Can you work these out from the model? Positions are in its coordinate system, mm. A direction names the side the tool comes from. Give positions to 0.01 mm unless a question says otherwise; leave off trailing zeros. Order: outer loops, then holes, each group sorted by start corner. A loop starts at its lowest first (then second) coordinate and runs counter-clockwise, first axis right, second up. Notation, with made-up numbers: (-28.5, 30.5) - (-21.5, 30.5) arc R7 cw to (-21.5, 37.5) - close; hole circle Ø8 at (17.5, -37.75). An arc over 180 degrees is marked (long way). Use one line per item in the form item = value. Start each with the question number.
1) We'd pull the mould along Y, two halves only. Please class faces 4 (the flat face through (-31.3, -1.7, 3)), 5 (the flat face through (-140.5, 83, 3)), 6 (the flat face through (-150, 86, 2)): released by +Y, released by -Y, zero draft, split by the parting line, or undercut.
2) Suppose I cut it at A-A, the plane z = 4.65. State how many separate pieces and enclosed holes the cut face has, and give its area (3 significant figures).
3) For pin 1 (3.5 mm diameter, centred on x = -30, y = -3, fed in from +Z); pin 2 (1 mm diameter, centred on x = -135, z = 1.5, fed in from -Y); pin 3 (3 mm diameter, centred on y = -4, z = 3, fed in from -X), each with a flat end and sliding along its axis, tell me the tip position at first contact or that it passes through.
4) Which directions (+Z, -Z, +X, -X, +Y, -Y) give clear straight access to the entire face, cutting with the end or side of a thin tool? Please do faces 1 (the flat face through (-20, -3, 3)), 2 (the flat face through (-40, -3, 3)), 3 (the flat face through (-269.7, 81.7, 3)).
5) Please list where these lines run through material, in increasing order: probe 1 along X at (y, z) = (83, 2.25); probe 2 along Y at (x, z) = (-150.5, 2); probe 3 along X at (y, z) = (82, 3.55).
6) Suppose I cut it at B-B, the plane x = -78.5. Write out the boundary of the cut face in (y, z), and give its area (3 significant figures).
```python
from build123d import *

# Parameters (mm, degrees)
BOSS_EXTRU_1_DEPTH      = 6
ESQUISSE2_R             = 1.5
ENL_V_MAT_EXTRU_1_DEPTH = 314.10221973
ESQUISSE3_R             = 2.995
ENL_V_MAT_EXTRU_2_DEPTH = 3


with BuildPart() as part:
    # Esquisse1 → Boss.-Extru.1 (new body)
    with BuildSketch(Plane.XY):
        Polygon((-40, 80), (-140.5, 80), (-140.5, 86), (-160.5, 86), (-160.5, 80), (-261, 80), (-261, 86), (-281, 86), (-281, 80), (-301, 80), (-301, 0), (-281, 0), (-281, -6), (-261, -6), (-261, 0), (-160.5, 0), (-160.5, -6), (-140.5, -6), (-140.5, 0), (-40, 0), (-40, -6), (-20, -6), (-20, 0), (0, 0), (0, 80), (-20, 80), (-20, 86), (-40, 86), align=None)
    extrude(amount=BOSS_EXTRU_1_DEPTH)

    # Esquisse2 → Enlèv. mat.-Extru.1 (cut, through all)
    with BuildSketch(Plane.XY.offset(6)):
        with Locations((-271, 83)):
            Circle(ESQUISSE2_R)
        with Locations((-150.5, 83)):
            Circle(ESQUISSE2_R)
        with Locations((-30, 83)):
            Circle(ESQUISSE2_R)
        with Locations(Location((-271, -3, 0), (0, 0, 180))):
            Circle(ESQUISSE2_R)
        with Locations(Location((-150.5, -3, 0), (0, 0, 180))):
            Circle(ESQUISSE2_R)
        with Locations(Location((-30, -3, 0), (0, 0, 180))):
            Circle(ESQUISSE2_R)
    extrude(amount=-ENL_V_MAT_EXTRU_1_DEPTH, mode=Mode.SUBTRACT)

    # Esquisse3 → Enlèv. mat.-Extru.2 (cut)
    with BuildSketch(Plane.XY.offset(6)):
        with Locations((-271, 83)):
            Circle(ESQUISSE3_R)
        with Locations((-150.5, 83)):
            Circle(ESQUISSE3_R)
        with Locations((-30, 83)):
            Circle(ESQUISSE3_R)
        with Locations(Location((-30, -3, 0), (0, 0, 180))):
            Circle(ESQUISSE3_R)
        with Locations(Location((-150.5, -3, 0), (0, 0, 180))):
            Circle(ESQUISSE3_R)
        with Locations(Location((-271, -3, 0), (0, 0, 180))):
            Circle(ESQUISSE3_R)
    extrude(amount=-ENL_V_MAT_EXTRU_2_DEPTH, mode=Mode.SUBTRACT)


solid = part.part
```
Result sheet:
q1.face_4 = undercut
q1.face_5 = zero draft
q1.face_6 = released by +Y
q2.separate_pieces = 1
q2.enclosed_holes = 6
q2.area = 24,600 mm²
q3.pin_1 = 3
q3.pin_2 = 0
q3.pin_3 = -281
q4.face_1 = +Z, -Z, +X, -Y
q4.face_2 = +Z, -Z, -Y
q4.face_3 = +Z
q5.probe_1 = -281 to -272.5, -269.5 to -261, -160.5 to -152, -149 to -140.5, -40 to -31.5, -28.5 to -20
q5.probe_2 = -6 to -4.5, -1.5 to 81.5, 84.5 to 86
q5.probe_3 = -281 to -273.82, -268.18 to -261, -160.5 to -153.32, -147.68 to -140.5, -40 to -32.82, -27.18 to -20
q6.outline = (0, 0) - (80, 0) - (80, 6) - (0, 6) - close
q6.area = 480 mm²
